Geometry: see drawing. Coordinates: mm, zero at the bounding-box minimum. Coordinates: 2 decimals unless noted, no trailing zeros. Loops run counter-clockwise (first coordinate to the right, second up) from the corner with the lowest first, then second, coordinate; pieces in that order, holes last. Notation, with made-up numbers: (-24, 88) -> (6, 88) arc R20 cw to (6, 110) -> close; hole circle Ø5 at (68, 72.25). An arc over 180 degrees is marked (long way). Answer as a JSON object with one key per item and string values.
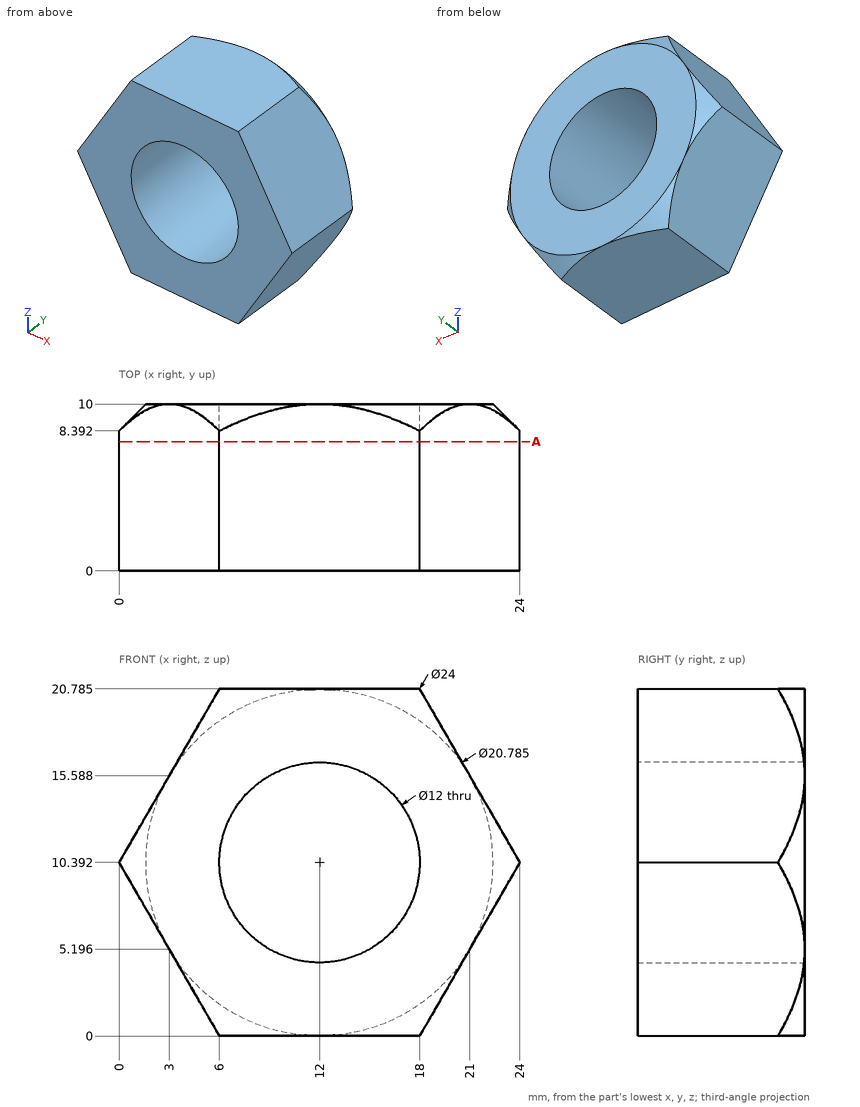
1. Pin query (flat end, axial travel): P1, Ø1.5, axis at x = 13.5, z = 5.5, coming from the +Y side; P2, Ø5, axis at y = 9, z = 2.5, coming from the -X side; P3, Ø1, axis at y = 5.5, z = 5.5, coming from the -X side (1 decimal); P4, Ø5, axis at y = 5, z = 10.5, coming from the +X side. Return the tip coordinate at first contact, or that it passes through.
Reply:
{"P1": "passes through", "P2": "stops at x = 3.11", "P3": "stops at x = 2.5", "P4": "stops at x = 24"}
2. Line query: line 1 along Z through (x, y) = (15.75, 4.75) (1 decimal); line 2 along Z through (x, y) = (8.5, 2) (1 decimal); line 3 along X through (y, z) = (8.5, 11.75) (1 decimal). Output: solid intervals per line, ascending.
Reply:
{"line 1": "z = 0 to 5.7, 15.1 to 20.8", "line 2": "z = 0 to 5.5, 15.3 to 20.8", "line 3": "x = 0.8 to 6.2, 17.8 to 23.2"}
3. Section query A-A (y = 7.75). Return loops of the section in (x, z) (1 decimal), plus the area to 3 significant figures.
Reply:
{"outline": "(0, 10.4) -> (6, 0) -> (18, 0) -> (24, 10.4) -> (18, 20.8) -> (6, 20.8) -> close; hole circle Ø12 at (12, 10.4)", "area": "261 mm2"}
